from build123d import *

# Parameters (mm, degrees)
F0_W     = 635
F0_H     = 38.1
F1_DEPTH = 1600
F2_W     = 372
F2_H     = 190
F3_DEPTH = 38.101
F4_R     = 88.9
F6_DEPTH = 38.101


with BuildPart() as f1:
    # F0 (on Right) → F1 (new body)
    with BuildSketch(Plane.YZ):
        with Locations((317.5, 19.05)):
            Rectangle(F0_W, F0_H)
    extrude(amount=F1_DEPTH)

    # F2 (on Top) → F3 (cut, through all)
    with BuildSketch(Plane.XY):
        with Locations((291, 540)):
            Rectangle(F2_W, F2_H)
    extrude(amount=F3_DEPTH, mode=Mode.SUBTRACT)

    # F4
    f4_edges = [f1.edges().sort_by_distance(p)[0] for p in [
        (477, 445, 19.05),
        (105, 445, 19.05),
    ]]
    fillet(f4_edges, radius=F4_R)

    # F5 (on Top) → F6 (cut, through all)
    with BuildSketch(Plane.XY):
        with BuildLine():
            Line((533.9, 105), (766.1, 105))
            ThreePointArc((766.1, 105), (828.961793, 131.038207), (855, 193.9))
            Line((855, 193.9), (855, 388.1))
            ThreePointArc((855, 388.1), (828.961793, 450.961793), (766.1, 477))
            Line((766.1, 477), (533.9, 477))
            ThreePointArc((533.9, 477), (471.038207, 450.961793), (445, 388.1))
            Line((445, 388.1), (445, 193.9))
            ThreePointArc((445, 193.9), (471.038207, 131.038207), (533.9, 105))
        make_face()
    extrude(amount=F6_DEPTH, mode=Mode.SUBTRACT)


solid = f1.part
CAD build for the part. Positions are in the model's coordinates, mm. A direction names the side the tool comes from. Round coordinates to 2 decimals unless told otherwise and drop trailing zeros. Write each loop counter-clockwise with the first axis right and the second up, starting at its lowest first coordinate (ties: lowest second). Pieces come first, ordered by that corner, then holes. Notation, with made-up numbers: M -7,-19.75 L 2,-19.75 A37 cw 2,16.25 Z; hole C 43.5,56.25 d7. An arc over 180 degrees is marked long. Put each result on its own line as item: value. Start each with the question number.
1) Saw through at D-D, the plane x = 269. Write the cut outline in (y, z), and give its area (3 significant figures).
2) Saw through at A-A, the plane x = 600. Write the cut outline in (y, z).
3) Saw through at B-B, the plane y = 298. Write the cut outline in (x, z).
4) Pin check, flat tip, straight feed: pin 1 Ø5 at (x, z) = (224, 32.5) entering from +Y. Stop position of the tip, or through.
5) 3-axis set-ups, long thin cutter, end or side, ignore diameter. For faces 1 (the cylindrical face through (450.267, 470.351, 19.317)), 2 (the cylindrical face through (470.351, 131.733, 18.783)), 3 (the flat face through (967, 313, 38.1)): which of +Z, -Z, +X, -X, +Y, -Y reach the whole face in a straight line?
6) Pull direction Y, two halves, no side cores. Call faces 4 (the flat face through (789, 0, 19)), 5 (the cylindrical face through (829.649, 450.267, 18.783)), 6 (the flat face through (290, 445, 19)), 7 (the flat face through (1600, 313, 19)): pulls with the +Y half, pulls with the -Y half, needs draft (parallel to the pull), parting line crosses it, or undercut.
7) Saw through at C-C, the plane z = 30. Write the cut outline in (x, y), and give its area (3 significant figures).
8) Drill centre lines: probe 1 along X at (y, z) = (284, 14.5); probe 2 along X at (y, z) = (581, 10.5); probe 3 along Y at (x, z) = (531.5, 35). Where is each one in solid material? Low to high. Write a range as [from, to].
Resolved:
1. outline: M 0,0 L 445,0 L 445,38.1 L 0,38.1 Z
1. area: 17,000 mm²
2. outline: M 0,0 L 105,0 L 105,38.1 L 0,38.1 Z; M 477,0 L 635,0 L 635,38.1 L 477,38.1 Z
3. outline: M 0,0 L 445,0 L 445,38.1 L 0,38.1 Z; M 855,0 L 1600,0 L 1600,38.1 L 855,38.1 Z
4. pin 1: y = 445
5. face 1: +Z, -Z, +Y
5. face 2: +Z, -Z
5. face 3: +Z, +X, -X, +Y, -Y
6. face 4: pulls with the -Y half
6. face 5: undercut
6. face 6: pulls with the +Y half
6. face 7: needs draft
7. outline: M 0,0 L 1600,0 L 1600,635 L 477,635 L 477,533.9 A88.9 cw 388.1,445 L 193.9,445 A88.9 cw 105,533.9 L 105,635 L 0,635 Z; hole M 445,193.9 A88.9 ccw 533.9,105 L 766.1,105 A88.9 ccw 855,193.9 L 855,388.1 A88.9 ccw 766.1,477 L 533.9,477 A88.9 ccw 445,388.1 Z
7. area: 803,000 mm²
8. probe 1: [0, 445], [855, 1600]
8. probe 2: [0, 105], [477, 1600]
8. probe 3: [0, 105.03], [476.97, 635]
